Model file for the job. Use its own axes, mm. Round coordinates to 2 decimals unless told otherwise and drop trailing zeros. Write each loop counter-clockwise with the first axis right and the second up, starting at its lowest first coordinate (ties: lowest second). Pieces come first, ordered by that corner, then holes.
```python
from build123d import *

# Parameters (mm, degrees)
BOSS_EXTRUDE1_DEPTH         = 50.8
F_1_4_28_TAPPED_HOLE1_D     = 5.4102
F_1_4_28_TAPPED_HOLE1_DEPTH = 57.15
F_1_4_28_TAPPED_HOLE1_TIP   = 1.625388061
F_1_4_28_TAPPED_HOLE2_D     = 5.4102
F_1_4_28_TAPPED_HOLE2_DEPTH = 57.15
F_1_4_28_TAPPED_HOLE2_TIP   = 1.625388061


with BuildPart() as part:
    # Sketch1 → Boss-Extrude1 (new, symmetric)
    with BuildSketch(Plane.XY):
        Polygon((7.332348419, 0), (3.666174209, 6.35), (-3.666174209, 6.35), (-7.332348419, 0), (-3.666174209, -6.35), (3.666174209, -6.35), align=None)
    extrude(amount=BOSS_EXTRUDE1_DEPTH, both=True)

    # 1/4-28 Tapped Hole1
    with Locations(Plane.XY.offset(50.8)):
        with Locations((0, 0)):
            Hole(F_1_4_28_TAPPED_HOLE1_D / 2, depth=F_1_4_28_TAPPED_HOLE1_DEPTH)
            with Locations((0, 0, -(F_1_4_28_TAPPED_HOLE1_DEPTH + F_1_4_28_TAPPED_HOLE1_TIP / 2))):  # 118° drill point
                Cone(0, F_1_4_28_TAPPED_HOLE1_D / 2, F_1_4_28_TAPPED_HOLE1_TIP, mode=Mode.SUBTRACT)

    # 1/4-28 Tapped Hole2
    with Locations(Plane(origin=(0, 0, -50.8), x_dir=(-1, 0, 0), z_dir=(0, 0, -1))):
        with Locations((0, 0)):
            Hole(F_1_4_28_TAPPED_HOLE2_D / 2, depth=F_1_4_28_TAPPED_HOLE2_DEPTH)
            with Locations((0, 0, -(F_1_4_28_TAPPED_HOLE2_DEPTH + F_1_4_28_TAPPED_HOLE2_TIP / 2))):  # 118° drill point
                Cone(0, F_1_4_28_TAPPED_HOLE2_D / 2, F_1_4_28_TAPPED_HOLE2_TIP, mode=Mode.SUBTRACT)


solid = part.part
```
1) Cut at B-B on x = 0. List the corners of the cut face in (y, z), and give its area (3 significant figures).
2) Cut at C-C on y = -1. List the corners of the cut face in (x, z) (3 decimals).
3) Wall check: probe 1 along X at (y, z) = (0, -27.5); probe 2 along Y at (x, z) = (0, 31.5); probe 3 along Y at (x, z) = (0.75, 3.5). Give the ranges that are in metal, low to high.
4) Cut at D-D on x = 5.25. List the corners of the cut face in (y, z), and give its area (3 significant figures).
5) Cut at A-A on z = -29.5. List the corners of the cut face in (x, y), and give its area (3 significant figures).
6) Flat gauge pins, fed straight in: pin 1 Ø3 at (y, z) = (2, -7) entering from +X; pin 2 Ø2 at (x, z) = (-5, -29) entering from -Y. Where does each tip first touch, or does it go through?
Result sheet:
1. outline: (-6.35, -50.8) - (-2.71, -50.8) - (-2.71, 50.8) - (-6.35, 50.8) - close; (2.71, -50.8) - (6.35, -50.8) - (6.35, 50.8) - (2.71, 50.8) - close
1. area: 741 mm2
2. outline: (-6.755, -50.8) - (-2.513, -50.8) - (-2.513, 50.8) - (-6.755, 50.8) - close; (2.513, -50.8) - (6.755, -50.8) - (6.755, 50.8) - (2.513, 50.8) - close
3. probe 1: x = -7.33 to -2.71, 2.71 to 7.33
3. probe 2: y = -6.35 to -2.71, 2.71 to 6.35
3. probe 3: y = -6.35 to -2.6, 2.6 to 6.35
4. outline: (-3.61, -50.8) - (3.61, -50.8) - (3.61, 50.8) - (-3.61, 50.8) - close
4. area: 733 mm2
5. outline: (-7.33, 0) - (-3.67, -6.35) - (3.67, -6.35) - (7.33, 0) - (3.67, 6.35) - (-3.67, 6.35) - close; hole circle Ø5.41 at (0, 0)
5. area: 117 mm2
6. pin 1: stops at x = 7.04
6. pin 2: stops at y = -5.77
